Work out the finished part from the listing and answer in its coordinate system (mm). Face numbers are marked on the shaded views. A direction names the side the tool comes from. Round coordinates to 2 decimals unless told otherwise and drop trailing zeros. Loops run counter-clockwise (first coordinate to the right, second up) from the corner with the lowest first, then second, coordinate; pieces in that order, holes last. Notation, with made-up numbers: (71.5, -35.75) -> (113.5, -35.75) arc R33 ccw to (113.5, -5.75) -> close; hole circle Ø6 at (-21.75, 52.25). An arc over 180 degrees is marked (long way). Use one line per item in the form item = value.
```python
from build123d import *

# Parameters (mm, degrees)
SKETCH1_W           = 15
SKETCH1_H           = 20
BOSS_EXTRUDE1_DEPTH = 3
SKETCH3_W           = 15
SKETCH3_H           = 3
BOSS_EXTRUDE3_DEPTH = 20
SKETCH4_R           = 3
CUT_EXTRUDE1_DEPTH  = 30.261749777
SKETCH2_R           = 3
CUT_EXTRUDE2_DEPTH  = 15
FILLET1_R           = 8


with BuildPart() as part:
    # Sketch1 → Boss-Extrude1 (new body)
    with BuildSketch(Plane(origin=(0, 0, 0), x_dir=(1, 0, 0), z_dir=(0, 1, 0))):
        Rectangle(SKETCH1_W, SKETCH1_H)
    extrude(amount=BOSS_EXTRUDE1_DEPTH)

    # Sketch3 → Boss-Extrude3 (add)
    with BuildSketch(Plane.XZ):
        with Locations((0, -8.5)):
            Rectangle(SKETCH3_W, SKETCH3_H)
        with Locations((0, 8.5)):
            Rectangle(SKETCH3_W, SKETCH3_H)
    extrude(amount=BOSS_EXTRUDE3_DEPTH)

    # Sketch4 → Cut-Extrude1 (cut, through all)
    with BuildSketch(Plane(origin=(0, 0, -10), x_dir=(-1, 0, 0), z_dir=(0, 0, -1))):
        with Locations((0, -12)):
            Circle(SKETCH4_R)
    extrude(amount=-CUT_EXTRUDE1_DEPTH, mode=Mode.SUBTRACT)

    # Sketch2 → Cut-Extrude2 (cut)
    with BuildSketch(Plane(origin=(0, 3, 0), x_dir=(1, 0, 0), z_dir=(0, 1, 0))):
        with Locations(Location((0, 0, 0), (0, 0, 270))):
            Circle(SKETCH2_R)
    extrude(amount=-CUT_EXTRUDE2_DEPTH, mode=Mode.SUBTRACT)

    # Fillet1
    # the kernel refuses this fillet: 8 mm, written as the material it takes off along each edge
    with BuildSketch(Plane(origin=(-7.5, -20, 30), x_dir=(0, 1, 0), z_dir=(0, 0, -1)), Plane(origin=(7.5, -20, -13), x_dir=(0, 1, 0), z_dir=(0, 0, 1))) as fillet1_piece_1:
        with BuildLine():
            CenterArc((FILLET1_R, FILLET1_R), FILLET1_R, 180, 90)
            Line((0, FILLET1_R), (0, 0))
            Line((0, 0), (FILLET1_R, 0))
        make_face()
    extrude(amount=43, mode=Mode.SUBTRACT)
    with BuildSketch(Plane(origin=(7.5, -20, 13), x_dir=(0, 1, 0), z_dir=(0, 0, -1)), Plane(origin=(-7.5, -20, -30), x_dir=(0, 1, 0), z_dir=(0, 0, 1))) as fillet1_piece_2:
        with BuildLine():
            CenterArc((FILLET1_R, -FILLET1_R), FILLET1_R, 90, 90)
            Line((0, -FILLET1_R), (0, 0))
            Line((0, 0), (FILLET1_R, 0))
        make_face()
    extrude(amount=43, mode=Mode.SUBTRACT)


solid = part.part
```
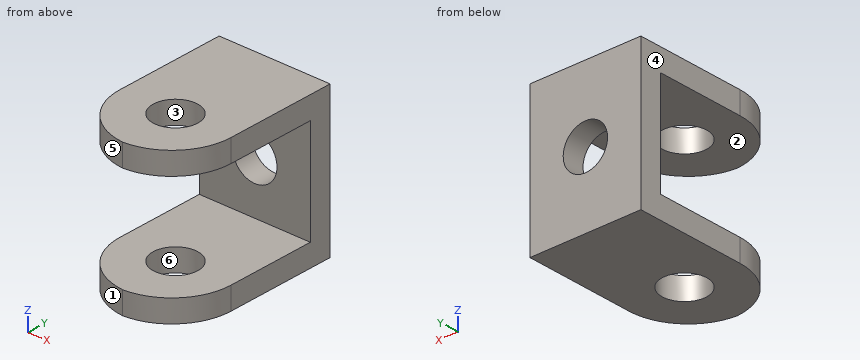
(1) For a pull along Y with two mould halves and no side action, classify the marked faces 3, 4, 5 and 6 as +Y half, -Y half, draft (parallel to the pull), parting line (faces both ways), or undercut.
Completed:
face_3 = undercut
face_4 = draft
face_5 = -Y half
face_6 = undercut
(2) Find section A-A, the plane y = -6. Write down the section's boundary in (x, z).
Completed:
outline = (-7.5, -10) -> (7.5, -10) -> (7.5, -7) -> (-7.5, -7) -> close; (-7.5, 7) -> (7.5, 7) -> (7.5, 10) -> (-7.5, 10) -> close
(3) Consider L1, parallel to Z at x = -4, y = -11; L2, parallel to Y at x = 0, z = 8.6; L3, parallel to Y at x = -5.5, z = 0.25. Determine where each line is inside the solid, lowest interval first.
Completed:
L1 = -10 to -7, 7 to 10
L2 = -19.98 to -15, -9 to 3
L3 = 0 to 3
(4) Given P1, Ø3.5, axis at x = 0, z = 0, coming from the -Y side; P2, Ø1.5, axis at x = -2, z = 3, coming from the -Y side, each flat-ended and moving along its own axis, determine where each tip first touches the part or whether it passes through.
Completed:
P1 = through
P2 = 0
(5) Find section D-D, the plane x = -5.25. Write down the section's boundary in (y, z).
Completed:
outline = (-17.56, -10) -> (3, -10) -> (3, 10) -> (-17.56, 10) -> (-17.56, 7) -> (0, 7) -> (0, -7) -> (-17.56, -7) -> close
(6) Find section C-C, the plane z = 0. Write down the section's boundary in (x, y).
Completed:
outline = (-7.5, 0) -> (-3, 0) -> (-3, 3) -> (-7.5, 3) -> close; (3, 0) -> (7.5, 0) -> (7.5, 3) -> (3, 3) -> close
(7) For the marked faces 1 and 2, determine the directions among +Z, -Z, +X, -X, +Y, -Y from which every point of the face is accessible in a straight line to the end or side of a thin tool.
Completed:
face_1 = +Z, -Z, -X, -Y
face_2 = +X, -X, -Y
(8) Find section B-B, the plane z = 8. Write down the section's boundary in (x, y).
Completed:
outline = (-7.5, -12) arc R8 ccw to (0, -19.98) arc R8 ccw to (7.5, -12) -> (7.5, 3) -> (-7.5, 3) -> close; hole circle Ø6 at (0, -12)
